The model under review builds one solid part; all positions refer to its coordinate system, in mm. A direction names the side the tool comes from. Give positions to 0.01 mm unless a question says otherwise; leave off trailing zeros. Order: outer loops, then holes, each group sorted by start corner. A loop starts at its lowest first (then second) coordinate and runs counter-clockwise, first axis right, second up. Notation, with made-up numbers: (7, 52) - (25, 52) arc R15 ccw to (25, 75) - close; hole circle Ø10 at (-16, 58.5). An arc over 180 degrees is marked (long way). Use a Markdown table: item, result. Add a question column.
```python
from build123d import *

# Parameters (mm, degrees)
SKETCH1_W           = 10
SKETCH1_H           = 37.8
SKETCH1_W_2         = 5.5
SKETCH1_H_2         = 3
BOSS_EXTRUDE1_DEPTH = 1
SKETCH2_W           = 10
SKETCH2_H           = 2
BOSS_EXTRUDE2_DEPTH = 4
BOSS_EXTRUDE3_START = -10.5
BOSS_EXTRUDE3_DEPTH = 3
BOSS_EXTRUDE4_START = 7.5
BOSS_EXTRUDE4_DEPTH = 3
FILLET1_R           = 0.8


with BuildPart() as part:
    # Sketch1 → Boss-Extrude1 (new, symmetric)
    with BuildSketch(Plane(origin=(0, 0, 0), x_dir=(1, 0, 0), z_dir=(0, 1, 0))):
        Rectangle(SKETCH1_W, SKETCH1_H)
        with Locations((-7.75, -17.4)):
            Rectangle(SKETCH1_W_2, SKETCH1_H_2)
        with Locations((7.75, -17.4)):
            Rectangle(SKETCH1_W_2, SKETCH1_H_2)
    extrude(amount=BOSS_EXTRUDE1_DEPTH, both=True)

    # Sketch2 → Boss-Extrude2 (add)
    with BuildSketch(Plane.XZ.offset(1)):
        with Locations((0, -17.9)):
            Rectangle(SKETCH2_W, SKETCH2_H)
    extrude(amount=BOSS_EXTRUDE2_DEPTH)

    # Sketch3 → Boss-Extrude3 (add)
    with BuildSketch(Plane(origin=(0, 0, 0), x_dir=(0, 0, -1), z_dir=(1, 0, 0)).offset(BOSS_EXTRUDE3_START)):
        with BuildLine():
            Line((-18.9, -7), (-22.9, -7))
            Line((-22.9, -7), (-22.9, -1))
            ThreePointArc((-22.9, -1), (-22.314213562, 0.414213562), (-20.9, 1))
            Line((-20.9, 1), (-18.9, 1))
            Line((-18.9, 1), (-18.9, -1))
            Line((-18.9, -1), (-19.9, -1))
            ThreePointArc((-19.9, -1), (-20.607106781, -1.292893219), (-20.9, -2))
            Line((-20.9, -2), (-20.9, -5))
            Line((-20.9, -5), (-17.9, -5))
            Line((-17.9, -5), (-17.9, -6))
            Line((-17.9, -6), (-18.9, -7))
        make_face()
    extrude(amount=BOSS_EXTRUDE3_DEPTH)

    # Sketch3<3> → Boss-Extrude4 (add)
    with BuildSketch(Plane(origin=(0, 0, 0), x_dir=(0, 0, -1), z_dir=(1, 0, 0)).offset(BOSS_EXTRUDE4_START)):
        with BuildLine():
            Line((-18.9, -7), (-22.9, -7))
            Line((-22.9, -7), (-22.9, -1))
            ThreePointArc((-22.9, -1), (-22.314213562, 0.414213562), (-20.9, 1))
            Line((-20.9, 1), (-18.9, 1))
            Line((-18.9, 1), (-18.9, -1))
            Line((-18.9, -1), (-19.9, -1))
            ThreePointArc((-19.9, -1), (-20.607106781, -1.292893219), (-20.9, -2))
            Line((-20.9, -2), (-20.9, -5))
            Line((-20.9, -5), (-17.9, -5))
            Line((-17.9, -5), (-17.9, -6))
            Line((-17.9, -6), (-18.9, -7))
        make_face()
    extrude(amount=BOSS_EXTRUDE4_DEPTH)

    # Fillet1
    fillet1_edges = [part.edges().sort_by_distance(p)[0] for p in [
        (0, -1, -16.9),
    ]]
    fillet(fillet1_edges, radius=FILLET1_R)


solid = part.part
```
Q1. Draft analysis for pull direction Y (two halves, no side actions). For faces 4 (the flat face through (-10.5, -3, 22)), 5 (the flat face through (9, -5, 19)), 6 (the flat face through (9, -6.5, 18.4)), state which applies: pulls with the +Y half, pulls with the -Y half, needs draft (parallel to the pull), parting line crosses it, or undercut.
Q2. We need section A-A (y = -3.25). Write out the cut boundary in (x, z).
Q3. Machinability: for faces 1 (the flat face through (-9, -5, 19)), 2 (the flat face through (8, 0, 15.9)), 3 (the flat face through (9, -5.5, 17.9)), which of the approach directions +Z, -Z, +X, -X, +Y, -Y give a long, thin tool a straight path to every point of the face, cutting with its end or side? Answer none if there is none.
Q4. We need section C-C (z = 16.5). Write out the cut boundary in (x, y), plus the area to 3 significant figures.
Q5. We need section D-D (x = 8). Write out the cut boundary in (y, z).
Q6. Wall thickness on probe 1 along X at (y, z) = (0, 20); probe 2 along Y at (x, z) = (-2, -13.5); probe 3 along Z at (x, y) = (3.75, -2.5): over which ranges is each line inside the solid? List them lowest first.
Q7. Clearance check with flat-ended pins moving along their axes: P1, Ø1.8, axis at y = -0.5, z = -2, coming from the +X side; P2, Ø2.5, axis at y = -3, z = 19.5, coming from the +X side; P3, Ø2.5, axis at x = 8.5, y = -3.5, coming from the -Z side; P4, Ø2, axis at x = 8.5, y = 0.5, coming from the -Z side. State where each tip first meets the part, or that it passes through.
Q8. We need section B-B (x = -1.25). Write out the cut boundary in (y, z), plus the area to 3 significant figures.
Here are the results:
| question | item | result |
|---|---|---|
| 1 | face 4 | needs draft |
| 1 | face 5 | undercut |
| 1 | face 6 | pulls with the -Y half |
| 2 | outline | (-10.5, 20.9) - (-7.5, 20.9) - (-7.5, 22.9) - (-10.5, 22.9) - close; (-5, -18.9) - (5, -18.9) - (5, -16.9) - (-5, -16.9) - close; (7.5, 20.9) - (10.5, 20.9) - (10.5, 22.9) - (7.5, 22.9) - close |
| 3 | face 1 | -Z, +X, -X |
| 3 | face 2 | -Z, +X, +Y, -Y |
| 3 | face 3 | -Z, +X, -X, -Y |
| 4 | outline | (-10.5, -1) - (10.5, -1) - (10.5, 1) - (-10.5, 1) - close |
| 4 | area | 42.0 mm2 |
| 5 | outline | (-7, 18.9) - (-6, 17.9) - (-5, 17.9) - (-5, 20.9) - (-2, 20.9) arc R1 cw to (-1, 19.9) - (-1, 15.9) - (1, 15.9) - (1, 20.9) arc R2 ccw to (-1, 22.9) - (-7, 22.9) - close |
| 6 | probe 1 | -10.5 to -7.5, 7.5 to 10.5 |
| 6 | probe 2 | -1 to 1 |
| 6 | probe 3 | -18.9 to -16.9 |
| 7 | P1 | x = 5 |
| 7 | P2 | through |
| 7 | P3 | z = 20.9 |
| 7 | P4 | z = 15.9 |
| 8 | outline | (-5, -18.9) - (1, -18.9) - (1, 18.9) - (-1, 18.9) - (-1, -16.1) arc R0.8 cw to (-1.8, -16.9) - (-5, -16.9) - close |
| 8 | area | 83.7 mm2 |
